from build123d import *

# Parameters (mm, degrees)
CYLINDER051_R             = 2.3
CYLINDER051_DEPTH         = 100
ARRAY001029_X_COUNT       = 2
ARRAY001029_X_PITCH       = 9
ARRAY001029_Z_COUNT       = 3
ARRAY001029_Z_PITCH       = 42.426407
CYLINDER048_R             = 2.3
CYLINDER048_DEPTH         = 100
ARRAY001026_Z_COUNT       = 2
ARRAY001026_Z_PITCH       = 9
BOX026_W                  = 20
BOX026_H                  = 3
BOX026_DEPTH              = 20
BOX026_PLACEMENT_ANGLE    = 45
BOX027_W                  = 20
BOX027_H                  = 3
BOX027_DEPTH              = 20
BOX027_PLACEMENT_ANGLE    = 45
BOX025_W                  = 28
BOX025_H                  = 3
BOX025_DEPTH              = 130
FUSION021_PLACEMENT_ANGLE = 45


with BuildPart() as horizontal_hole_array003:
    # Cylinder051 → Cylinder051 (new body)
    with BuildSketch(Plane(origin=(4, -10, 5), x_dir=(1, 0, 0), z_dir=(0, 1, 0))):
        Circle(CYLINDER051_R)
    extrude(amount=CYLINDER051_DEPTH)

    # Array001029 X: horizontal hole array003 ×2


with BuildPart() as horizontal_hole_array003_1:
    add(horizontal_hole_array003.part)
    with Locations(*[(i * ARRAY001029_X_PITCH, 0, 0) for i in range(1, ARRAY001029_X_COUNT)]):
        add(horizontal_hole_array003.part)

    # Array001029 Z: horizontal hole array003 ×3


with BuildPart() as horizontal_hole_array003_2:
    add(horizontal_hole_array003_1.part)
    with Locations(*[Vector(0.707107, 0, 0.707107) * (i * ARRAY001029_Z_PITCH) for i in range(1, ARRAY001029_Z_COUNT)]):
        add(horizontal_hole_array003_1.part)


with BuildPart() as horizontal_hole_array003_3:
    # Array001029 placement: moved
    add(horizontal_hole_array003_2.part.moved(Location((-98, 0, -86))))


with BuildPart() as fusion024:
    # Cylinder048 → Cylinder048 (new body)
    with BuildSketch(Plane(origin=(0, -10, 6), x_dir=(1, 0, 0), z_dir=(0, 1, 0))):
        Circle(CYLINDER048_R)
    extrude(amount=CYLINDER048_DEPTH)

    # Array001026 Z: Fusion024 ×2


with BuildPart() as fusion024_1:
    add(fusion024.part)
    with Locations(*[(0, 0, i * ARRAY001026_Z_PITCH) for i in range(1, ARRAY001026_Z_COUNT)]):
        add(fusion024.part)

    # Fusion024: union horizontal hole array003
    add(horizontal_hole_array003_3.part)


with BuildPart() as side_cube:
    # Box026 → Box026 (new body)
    with BuildSketch(Plane.XY):
        with Locations((10, 1.5)):
            Rectangle(BOX026_W, BOX026_H)
    extrude(amount=BOX026_DEPTH)


with BuildPart() as side_cube_1:
    # Box026 placement: moved
    add(side_cube.part.moved(Location((0, 0, 130))).rotate(Axis((0, 0, 130), (0, 1, 0)), BOX026_PLACEMENT_ANGLE))


with BuildPart() as side_cube001:
    # Box027 → Box027 (new body)
    with BuildSketch(Plane.XY):
        with Locations((10, 1.5)):
            Rectangle(BOX027_W, BOX027_H)
    extrude(amount=BOX027_DEPTH)


with BuildPart() as side_cube001_1:
    # Box027 placement: moved
    add(side_cube001.part.rotate(Axis((0, 0, 0), (0, 1, 0)), BOX027_PLACEMENT_ANGLE))


with BuildPart() as stand_attachment_side_plate_cut:
    # Box025 → Box025 (new body)
    with BuildSketch(Plane.XY):
        with Locations((14, 1.5)):
            Rectangle(BOX025_W, BOX025_H)
    extrude(amount=BOX025_DEPTH)

    # Fusion021: union side cube, side cube001
    add(side_cube_1.part)
    add(side_cube001_1.part)


with BuildPart() as stand_attachment_side_plate_cut_1:
    # Fusion021 placement: moved
    add(stand_attachment_side_plate_cut.part.moved(Location((-99.702056, -3, -71.417785))).rotate(Axis((-99.702056, -3, -71.417785), (0, 1, 0)), FUSION021_PLACEMENT_ANGLE))

    # Cut019: cut Fusion024
    add(fusion024_1.part, mode=Mode.SUBTRACT)


solid = stand_attachment_side_plate_cut_1.part
Here's how the part is built. I have some questions about the finished solid (model axes, mm). Give positions to 0.01 mm unless a question says otherwise; leave off trailing zeros. Loops run counter-clockwise (first coordinate to the right, second up) from the corner with the lowest first, then second, coordinate; pieces in that order, holes last. Notation, with made-up numbers: (-7.75, 24) -> (9.25, 24) arc R32 cw to (9.25, 57) -> close; hole circle Ø4 at (18.5, -39.75). An arc over 180 degrees is marked (long way). One line per item, written item: value.
Q1. I'm going to push a flat-ended pin straight in: pin 1 Ø1 at (y, z) = (-1.5, -7) entering from -X. Where does the tip first touch, or does it pass through?
Answers follow:
pin 1: x = -35.78
Q2. Suppose I cut it at A-A on z = 15. Please give me the cut outline in (x, y).
Answers follow:
outline: (-13.28, -3) -> (-2.3, -3) -> (-2.3, 0) -> (-13.28, 0) -> close; (2.3, -3) -> (12.22, -3) -> (12.22, 0) -> (2.3, 0) -> close
Q3. We'd pull the mould along Z, two halves only. Please class faces 1 (the face through (-99.702, -1, -81)), 2 (the face through (-34.582, -1.521, -45.895)), 3 (the face through (-95.825, -1.521, -79.6)), 4 (the face through (2, -2, 20.506)): pulls with the +Z half, pulls with the -Z half, needs draft (parallel to the pull), parting line crosses it, or undercut.
Answers follow:
face 1: needs draft
face 2: pulls with the -Z half
face 3: undercut
face 4: pulls with the +Z half
Q4. Suppose I cut it at B-B on x = -63.5. Please give me the cut outline in (y, z) (3 decimals).
Answers follow:
outline: (-3, -74.814) -> (0, -74.814) -> (0, -53.245) -> (-3, -53.245) -> close; (-3, -48.755) -> (0, -48.755) -> (0, -35.216) -> (-3, -35.216) -> close
Q5. Suppose I cut it at C-C on x = 0. Please give me the cut outline in (y, z).
Answers follow:
outline: (-3, -11.31) -> (0, -11.31) -> (0, 3.7) -> (-3, 3.7) -> close; (-3, 8.3) -> (0, 8.3) -> (0, 12.7) -> (-3, 12.7) -> close; (-3, 17.3) -> (0, 17.3) -> (0, 20.51) -> (-3, 20.51) -> close
Q6. If I drill on line 1 along X through (y, z) = (-2.6, -20.5); line 2 along X through (y, z) = (-0.4, -79.5); line 3 along Z through (x, y) = (-94, -1.45), over which ranges is the centre line in solid material (lowest first)?
Answers follow:
line 1: -48.78 to -36.24, -31.75 to -27.24, -22.75 to -9.19
line 2: -99.7 to -95.74, -92.26 to -86.74, -83.26 to -68.19
line 3: -91.42 to -83.3, -78.7 to -65.72
Q7. Suppose I cut it at D-D on y = -1.55. State how many separate pieces and enclosed holes the cut face has, then the cut area to 3 significant figures.
Answers follow:
separate pieces: 1
enclosed holes: 8
area: 3,910 mm^2
